Autodesk Inventor part; units mm, degrees
ref_plane "YZ Plane" through (0, 0, 0) normal (1, 0, 0) x (0, 1, 0)
ref_plane "XZ Plane" through (0, 0, 0) normal (0, 1, 0) x (-1, 0, 0)
ref_plane "XY Plane" through (0, 0, 0) normal (0, 0, 1) x (1, 0, 0)
sketch "Sketch3" plane through (0, 0, 0) normal (0, 0, 1) x (1, 0, 0)
  line L0 (0, 0) -> (65, 0)
  line L1 (65, 0) -> (65, 95)
  line L2 (65, 95) -> (57, 95)
  line L3 (57, 95) -> (57, 8)
  line L4 (57, 8) -> (0, 8)
  line L5 (0, 8) -> (0, 0)
  dimension "d17" = 8
  dimension "d18" = 57
  dimension "d19" = 87
  dimension "d20" = 8
extrude "Extrusion3" add sketch "Sketch3" against normal mid plane 16
sketch "Sketch5" plane through (0, 8, -8) normal (0, 1, 0) x (1, 0, 0)
  line L0 (-13, -8) -> (78, -8)
  circle A0 centre (10, -8) radius 1.9
  circle A1 centre (30, -8) radius 1.9
  line L1 (0, 0) -> (0, -16)
  point P0 (0, -8)
  dimension "d23" = 3.8
  dimension "d24" = 3.8
  dimension "d25" = 10
  dimension "d26" = 20
extrude "Extrusion4" cut sketch "Sketch5" against normal through all
chamfer "Chamfer2" distance 5 angle 45 1 edges at (0, 0, 0)
chamfer "Chamfer3" distance 10 angle 45 1 edges at (57, 8, 0)
chamfer "Chamfer4" distance 10 angle 45 1 edges at (65, 0, 0)
sketch "Sketch6" plane through (65, 95, 8) normal (1, 0, 0) x (0, 0, -1)
  line L0 (16, -77) -> (16, 0)
  line L1 (0, -85) -> (0, 0)
  circle A0 centre (8, -8) radius 8
  line L2 (16, 0) -> (0, 0)
  point P0 (8, -95)
  dimension "d39" = 16
extrude "Extrusion5" add sketch "Sketch6" along normal blind 7 contours A0
fillet "Fillet1" radius 8 2 edges at (61, 95, -8) (61, 95, 8)
sketch "Sketch7" plane through (57, 18, -8) normal (-1, 0, 0) x (0, 0, 1)
  point P0 (8, -18)
sketch "Sketch8" plane through (72, 87, 0) normal (1, 0, 0) x (0, 0, -1)
  circle A0 centre (0, 0) radius 8
  circle A1 centre (0, 0) radius 2.75
  point P0 (0, -87)
  dimension "d43" = 5.5
extrude "Extrusion6" add sketch "Sketch8" along normal blind 4 contours A1
sketch "Sketch9" plane through (76, 87, 0) normal (1, 0, 0) x (0, 0, -1)
  circle A0 centre (0, 0) radius 2.75 construction
  circle A1 centre (0, 0) radius 2.25
  point P0 (0, -87)
  dimension "d46" = 4.5
extrude "Extrusion7" cut sketch "Sketch9" against normal through all
sketch "Sketch10" plane through (57, 18, -8) normal (-1, 0, 0) x (0, 0, 1)
  circle A0 centre (8, 69) radius 2.25
  circle A1 centre (8, 69) radius 4.5
  point P0 (8, -18)
  dimension "d49" = 9
extrude "Extrusion8" cut sketch "Sketch10" against normal blind 3
chamfer "Chamfer5" distance 3 angle 45 1 edges at (57, 87, -4.5)
chamfer "Chamfer6" distance 3 angle 45 1 edges at (72, 87, 2.75)
sketch "Sketch11" plane through (76, 87, 0) normal (1, 0, 0) x (0, 0, -1)
  circle A0 centre (0, 0) radius 2.25
  circle A1 centre (0, 0) radius 10.166
  point P0 (0, -87)
extrude "Extrusion9" cut sketch "Sketch11" against normal blind 5
chamfer "Chamfer7" distance 4 angle 45 1 edges at (71, 87, 8)
equation "\"d20\" = d17"
properties part number "LinearActuatorToBottomPlateAdapter"
Geometry: final body of the model. Coordinates: model frame, mm. A direction names the side the tool comes from. Coordinates: 2 decimals unless noted, no trailing zeros. Write each loop counter-clockwise with the first axis right and the second up, starting at its lowest first coordinate (ties: lowest second). Pieces come first, ordered by that corner, then holes. Notation, with made-up numbers: (73.5, -7) - (82.5, -7) arc R28 ccw to (82.5, 31) - close; hole circle Ø11 at (18, 46.5). An arc over 180 degrees is marked (long way). Return JSON: item names as keys, results as strings.
Item 1: Section query D-D (x = 23). Output: boundary loops of the cut face in (y, z), and give its area (3 significant figures).
Completed:
{"outline": "(0, -8) - (8, -8) - (8, 8) - (0, 8) - close", "area": "128 mm2"}
Item 2: Pin query (flat end, axial travel): pin 1 Ø4 at (y, z) = (34.5, -3.5) entering from -X; pin 2 Ø4.5 at (y, z) = (87, -2) entering from -X; pin 3 Ø3 at (x, z) = (46.5, 4) entering from -Y; pin 4 Ø3 at (x, z) = (10.5, -0.5) entering from +Y. Return the tip coordinate at first contact, or that it passes through.
Completed:
{"pin 1": "stops at x = 57", "pin 2": "stops at x = 60", "pin 3": "stops at y = 0", "pin 4": "stops at y = 8"}
Item 3: Line query: L1, parallel to Z at x = 10, y = 3; L2, parallel to X at y = 4.25, z = 0; L3, parallel to X at y = 2.75, z = 0. Output: solid intervals per line, ascending.
Completed:
{"L1": "z = -8 to -1.9, 1.9 to 8", "L2": "x = 0.75 to 8.1, 11.9 to 28.1, 31.9 to 59.25", "L3": "x = 2.25 to 8.1, 11.9 to 28.1, 31.9 to 57.75"}
Item 4: Pull-direction query (Z, two-part tool) for faces 4 (the face through (71, 85, -2)), 5 (the face through (11.755, 4.056, 0.728)), 6 (the face through (60.944, 92.594, 5.719)); classes: +Z half, -Z half, draft (parallel to the pull), parting line (faces both ways), or undercut.
Completed:
{"face 4": "draft", "face 5": "undercut", "face 6": "+Z half"}
Item 5: Section query C-C (y = 47.5). Output: boundary loops of the cut face in (x, z).
Completed:
{"outline": "(57, -8) - (65, -8) - (65, 8) - (57, 8) - close"}
Item 6: Section query A-A (x = 10). Output: boundary loops of the cut face in (y, z).
Completed:
{"outline": "(0, -8) - (8, -8) - (8, -1.9) - (0, -1.9) - close; (0, 1.9) - (8, 1.9) - (8, 8) - (0, 8) - close"}
Item 7: Reachability of faces 1 (the face through (24, 8, 0)), 2 (the face through (60, 85, 2)), 3 (the face through (65.986, 79.068, 1.041)) from +Z, -Z, +X, -X, +Y, -Y: full face, straight path, thin tool, end or side. Return the list, or none.
Completed:
{"face 1": "+Z, -Z, -X, +Y", "face 2": "-X", "face 3": "+X"}
